Autodesk Inventor part; units mm, degrees
ref_plane "YZ Plane" through (0, 0, 0) normal (1, 0, 0) x (0, 1, 0)
ref_plane "XZ Plane" through (0, 0, 0) normal (0, 1, 0) x (-1, 0, 0)
ref_plane "XY Plane" through (0, 0, 0) normal (0, 0, 1) x (1, 0, 0)
sketch "Sketch1" plane through (0, 0, 0) normal (0, 1, 0) x (-1, 0, 0)
  line L0 (16.7626, -83.8715) -> (19.7626, -83.8715)
  line L1 (19.7626, -83.8715) -> (19.7626, -85.3715)
  line L2 (19.7626, -85.3715) -> (10.7873, -88.3968)
  line L3 (10.7873, -88.3968) -> (7.7622, -97.3718)
  line L4 (7.7622, -97.3718) -> (6.2622, -97.3718)
  line L5 (6.2622, -97.3718) -> (6.2622, -94.3718)
  line L6 (6.2622, -94.3718) -> (7.2622, -94.3718)
  line L7 (7.2622, -94.3718) -> (7.2622, -90.3718)
  line L8 (7.2622, -90.3718) -> (3.2622, -90.3718)
  line L9 (3.2622, -90.3718) -> (3.2622, -94.3718)
  line L10 (3.2622, -94.3718) -> (4.2622, -94.3718)
  line L11 (4.2622, -94.3718) -> (4.2622, -97.3718)
  line L12 (4.2622, -97.3718) -> (2.7622, -97.3718)
  line L13 (2.7622, -97.3718) -> (-1.3715, -85.1077)
  arc A0 (7.4979, -76.2381) -> (-1.3715, -85.1077) centre (5.2622, -82.8718) ccw
  line L14 (7.4979, -76.2381) -> (19.7626, -80.3715)
  line L15 (19.7626, -80.3715) -> (19.7626, -81.8715)
  line L16 (19.7626, -81.8715) -> (16.7626, -81.8715)
  line L17 (16.7626, -81.8715) -> (16.7626, -80.8715)
  line L18 (16.7626, -80.8715) -> (12.7626, -80.8715)
  line L19 (12.7626, -80.8715) -> (12.7626, -84.8715)
  line L20 (12.7626, -84.8715) -> (16.7626, -84.8715)
  line L21 (16.7626, -84.8715) -> (16.7626, -83.8715)
  line L22 (6.3619, -198.0335) -> (6.3619, -195.0335)
  line L23 (6.3619, -195.0335) -> (7.8619, -195.0335)
  line L24 (7.8619, -195.0335) -> (10.8872, -204.0087)
  line L25 (10.8872, -204.0087) -> (19.8622, -207.0338)
  line L26 (19.8622, -207.0338) -> (19.8622, -208.5338)
  line L27 (19.8622, -208.5338) -> (16.8622, -208.5338)
  line L28 (16.8622, -208.5338) -> (16.8622, -207.5338)
  line L29 (16.8622, -207.5338) -> (12.8622, -207.5338)
  line L30 (12.8622, -207.5338) -> (12.8622, -211.5338)
  line L31 (12.8622, -211.5338) -> (16.8622, -211.5338)
  line L32 (16.8622, -211.5338) -> (16.8622, -210.5338)
  line L33 (16.8622, -210.5338) -> (19.8622, -210.5338)
  line L34 (19.8622, -210.5338) -> (19.8622, -212.0338)
  line L35 (19.8622, -212.0338) -> (7.5981, -216.1675)
  arc A1 (-1.2715, -207.2981) -> (7.5981, -216.1675) centre (5.3622, -209.5338) ccw
  line L36 (-1.2715, -207.2981) -> (2.8619, -195.0335)
  line L37 (2.8619, -195.0335) -> (4.3619, -195.0335)
  line L38 (4.3619, -195.0335) -> (4.3619, -198.0335)
  line L39 (4.3619, -198.0335) -> (3.3619, -198.0335)
  line L40 (3.3619, -198.0335) -> (3.3619, -202.0335)
  line L41 (3.3619, -202.0335) -> (7.3619, -202.0335)
  line L42 (7.3619, -202.0335) -> (7.3619, -198.0335)
  line L43 (7.3619, -198.0335) -> (6.3619, -198.0335)
  line L44 (2.7622, -97.3718) -> (2.8619, -195.0335)
  line L45 (7.8619, -195.0335) -> (7.7622, -97.3718)
  line L46 (2.812, -146.2026) -> (7.812, -146.2026)
  circle A2 centre (5.312, -146.2026) radius 4.5
  circle A3 centre (5.312, -146.2026) radius 7.5
  point P0 (0, 0)
  point P1 (7.8048, -139.129)
  point P2 (2.8048, -139.1341)
  point P3 (2.8193, -153.2762)
  point P4 (7.8193, -153.2711)
  dimension "d8" = 9
  dimension "d9" = 15
extrude "Extrusion1" add sketch "Sketch1" along normal blind 10 contours L45 A3 L44 L12 L11 L10 L9 L8 L7 L6 L5 L4 | A3 L45 A2 | L45 A2 L44 A3 | L44 A2 A3 | A3 L44 A2 L45 | L45 L23 L22 L43 L42 L41 L40 L39 L38 L37 L44 A3
sketch "Sketch2" plane through (0, 0, 0) normal (0, -1, 0) x (1, 0, 0)
  line L0 (-4.3619, -198.0335) -> (-3.3619, -198.0335)
  line L1 (-4.3619, -195.0335) -> (-4.3619, -198.0335)
  line L2 (-2.8619, -195.0335) -> (-4.3619, -195.0335)
  line L3 (-2.7622, -97.3718) -> (-2.8619, -195.0335)
  line L4 (-4.2622, -97.3718) -> (-2.7622, -97.3718)
  line L5 (-4.2622, -94.3718) -> (-4.2622, -97.3718)
  line L6 (-3.2622, -94.3718) -> (-4.2622, -94.3718)
  line L7 (-3.2622, -90.3718) -> (-3.2622, -94.3718)
  line L8 (-7.2622, -90.3718) -> (-3.2622, -90.3718)
  line L9 (-7.2622, -94.3718) -> (-7.2622, -90.3718)
  line L10 (-6.2622, -94.3718) -> (-7.2622, -94.3718)
  line L11 (-6.2622, -97.3718) -> (-6.2622, -94.3718)
  line L12 (-7.7622, -97.3718) -> (-6.2622, -97.3718)
  line L13 (-7.8619, -195.0335) -> (-7.7622, -97.3718)
  line L14 (-6.3619, -195.0335) -> (-7.8619, -195.0335)
  line L15 (-6.3619, -198.0335) -> (-6.3619, -195.0335)
  line L16 (-7.3619, -198.0335) -> (-6.3619, -198.0335)
  line L17 (-7.3619, -202.0335) -> (-7.3619, -198.0335)
  line L18 (-3.3619, -202.0335) -> (-7.3619, -202.0335)
  line L19 (-3.3619, -198.0335) -> (-3.3619, -202.0335)
  line L20 (-7.812, -146.2026) -> (-2.812, -146.2026)
  line L21 (-6.2622, -97.3718) -> (-4.2622, -97.3718)
  line L22 (-5.312, -146.2026) -> (-5.312, -121.2026)
  line L23 (-5.312, -146.2026) -> (-5.312, -171.2026)
  circle A0 centre (-5.312, -171.2026) radius 8
  circle A1 centre (-5.312, -121.2026) radius 8
  point P0 (0, 0)
  dimension "d2" = 25
  dimension "d3" = 25
  dimension "d4" = 16
  dimension "d5" = 16
extrude "Extrusion2" add sketch "Sketch2" along normal mid plane 20 contours A0 L13 L3 | L3 A0 | A0 L13 | A1 L13 L3 | L3 A1 | A1 L13
sketch "Sketch3" plane through (-5.312, -10, -121.2026) normal (0, -1, 0) x (1, 0, 0)
  circle A0 centre (0, 0) radius 8
  circle A1 centre (0, -50) radius 8
  circle A2 centre (0, 0) radius 5
  circle A3 centre (0, -50) radius 5
  point P0 (5.312, 121.2026)
  dimension "d10" = 10
extrude "Extrusion3" cut sketch "Sketch3" against normal blind 18 contours A2 | A3
properties part number "Leg_rod"
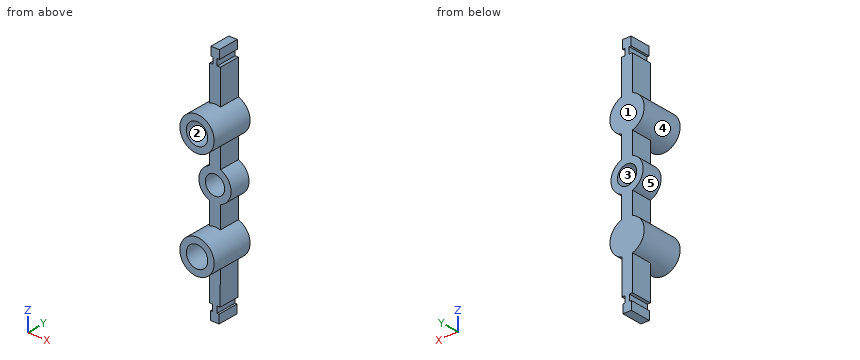
Geometry: final body of the model. Coordinates: model frame, mm. Face numbers are marked on the shaded views. A direction names the side the tool comes from. Round coordinates to 2 decimals unless told otherwise and drop trailing zeros. Loops run counter-clockwise (first coordinate to the right, second up) from the corner with the lowest first, then second, coordinate; pieces in that order, holes last. Notation, with made-up numbers: (3.25, 45) -> (21.25, 45) arc R24 cw to (21.25, 79) -> close; hole circle Ø3 at (-10.5, -7). An arc over 180 degrees is marked (long way). Use one line per item in the form item = value.
Item 1: Access query for the marked faces 1 and 2. Directions: +Z, -Z, +X, -X, +Y, -Y. A direction counts if a zero-diameter tool reaches every point of the face in a straight line with its end or side. Return the directions, or none.
Evaluation:
face_1 = +Z, -Z, +X, -X, +Y
face_2 = -Y
Item 2: Cut plane C-C on y = -8. Output: boundary loops of the cut face in (x, z), then the cut area to 3 significant figures.
Evaluation:
outline = circle Ø16 at (-5.31, -171.2); circle Ø16 at (-5.31, -121.2); hole circle Ø10 at (-5.31, -171.2); hole circle Ø10 at (-5.31, -121.2)
area = 245 mm2
Item 3: Contact query for flat-ended pins moving along their axis: pin 1 Ø4.5 at (x, z) = (-6, -154) entering from -Y; pin 2 Ø3.5 at (y, z) = (6.5, -197) entering from -X; pin 3 Ø1.2 at (y, z) = (4, -93.5) entering from -X. Output: stop coordinate, or through.
Evaluation:
pin_1 = 0
pin_2 = -7.36
pin_3 = -7.26
Item 4: Draft query along X for the marked faces 3, 4 and 5. Return one class per face: released by +X, released by -X, zero draft, split by the parting line, or undercut.
Evaluation:
face_3 = undercut
face_4 = split by the parting line
face_5 = released by -X
Item 5: Cut plane D-D on x = -11.25. Output: boundary loops of the cut face in (y, z), then the cut area to 3 significant figures.
Evaluation:
outline = (-10, -176.56) -> (10, -176.56) -> (10, -165.84) -> (-10, -165.84) -> close; (-10, -126.56) -> (10, -126.56) -> (10, -115.84) -> (-10, -115.84) -> close; (0, -150.78) -> (10, -150.78) -> (10, -141.62) -> (0, -141.62) -> close
area = 521 mm2
Item 6: Cut plane A-A on x = 1. Output: boundary loops of the cut face in (y, z).
Evaluation:
outline = (-10, -176.12) -> (10, -176.12) -> (10, -166.29) -> (-10, -166.29) -> close; (-10, -126.12) -> (10, -126.12) -> (10, -116.29) -> (-10, -116.29) -> close; (0, -150.25) -> (10, -150.25) -> (10, -142.15) -> (0, -142.15) -> close
Item 7: Material intervals for probe 1 along Z at (x, y) = (-5, -0.25); probe 2 along Z at (x, y) = (-5, 3.75); probe 3 along Z at (x, y) = (-3.5, 5.75), sorted ascending.
Evaluation:
probe_1 = -179.2 to -176.19, -166.21 to -163.21, -129.2 to -126.19, -116.21 to -113.21
probe_2 = -202.03 to -176.19, -166.21 to -150.69, -141.71 to -126.19, -116.21 to -90.37
probe_3 = -202.03 to -198.03, -195.03 to -175.86, -166.54 to -150.32, -142.08 to -125.86, -116.54 to -97.37, -94.37 to -90.37
Item 8: Cut plane B-B on z = -147.5. Output: boundary loops of the cut face in (x, y), then the cut area to 3 significant figures.
Evaluation:
outline = (-12.7, 0) -> (-9.62, 0) -> (-9.62, 10) -> (-12.7, 10) -> close; (-1, 0) -> (2.07, 0) -> (2.07, 10) -> (-1, 10) -> close
area = 61.6 mm2
